Here's how the part is built. I have some questions about the finished solid (model axes, mm). A direction names the side the tool comes from. Coordinates: 2 decimals unless noted, no trailing zeros. Loops run counter-clockwise (first coordinate to the right, second up) from the corner with the lowest first, then second, coordinate; pieces in that order, holes last. Notation, with made-up numbers: M 64,84.25 L 84,84.25 A7 cw 84,94.25 Z; hole C -11,70.5 d2. An arc over 180 degrees is marked long. Use CSV: the item, a comma, the result in double quotes. Start each with the question number.
Q1. If we section it at A-A (z = 0): Please give me the cut outline in (x, y), and give its area (3 significant figures).
Q2. Which directions (+Z, -Z, +X, -X, +Y, -Y) give clear straight access to the entire face, cutting with the end or side of a thin tool? Please do faces 4 (the cylindrical face through (-14, 1, 0)), 5 (the flat face through (-13.67, 4.08, 7.9)), 6 (the flat face through (13.84, 4.08, 7.79)), 7 (the cylindrical face through (0, 4, -14)), 8 (the flat face through (-20, 4, 3)).
Q3. If we mould it in two halves opening along X, with no side actions, what happens to faces 1 (the cylindrical face through (16.05, 4.08, -0.08)), 2 (the flat face through (20, 4, -3)), 3 (the flat face through (-4, 0, -5))? For each: +X half, -X half, draft (parallel to the pull), parting line (faces both ways), or undercut.
Q4. If we section it at D-D (y = 1.05): Please give me the cut outline in (x, z), and give its area (3 significant figures).
Q5. For pin 1 Ø6 at (x, z) = (15.5, 15.5) entering from +Y, with a flat end and sliding along its axis, tell me the tip position at first contact or that it passes through.
Q6. If we section it at C-C (y = 3.65): Please give me the cut outline in (x, z), and give its area (3 significant figures).
Q7. Please list where these lines run through material, in increasing order: probe 1 along Z at (x, y) = (17, 1.3); probe 2 along Y at (x, z) = (-13.5, 15.5); probe 3 along Z at (x, y) = (2, 2.2). Write a range as [from, to].
Q8. If we section it at B-B (x = 0): Please give me the cut outline in (y, z), and give its area (3 significant figures).
from build123d import *

# Parameters (mm, degrees)
SKETCH_1_R          = 1.8
SKETCH_1_R_2        = 5
EXTRUDE_1_DEPTH     = 3
EXTRUDE_2_DEPTH     = 2.2
SKETCH_3_R          = 5
CUT_EXTRUDE_1_DEPTH = 2.2


with BuildPart() as part:
    # 草图1 → 凸台-拉伸1 (new body)
    with BuildSketch(Plane(origin=(0, 0, 0), x_dir=(1, 0, 0), z_dir=(0, 1, 0))):
        with BuildLine():
            Line((20, -3.872983346), (20, -15))
            ThreePointArc((20, -15), (18.535533906, -18.535533906), (15, -20))
            Line((15, -20), (-15, -20))
            ThreePointArc((-15, -20), (-18.535533906, -18.535533906), (-20, -15))
            Line((-20, -15), (-20, -3.872983346))
            ThreePointArc((-20, -3.872983346), (-14, 0), (-20, 3.872983346))
            Line((-20, 3.872983346), (-20, 15))
            ThreePointArc((-20, 15), (-18.535533906, 18.535533906), (-15, 20))
            Line((-15, 20), (15, 20))
            ThreePointArc((15, 20), (18.535533906, 18.535533906), (20, 15))
            Line((20, 15), (20, 3.872983346))
            ThreePointArc((20, 3.872983346), (14, 0), (20, -3.872983346))
        make_face()
        with Locations((-15.5, 15.5)):
            Circle(SKETCH_1_R, mode=Mode.SUBTRACT)
        with Locations((15.5, 15.5)):
            Circle(SKETCH_1_R, mode=Mode.SUBTRACT)
        with Locations((-15.5, -15.5)):
            Circle(SKETCH_1_R, mode=Mode.SUBTRACT)
        with Locations((15.5, -15.5)):
            Circle(SKETCH_1_R, mode=Mode.SUBTRACT)
        Circle(SKETCH_1_R_2, mode=Mode.SUBTRACT)
    extrude(amount=EXTRUDE_1_DEPTH)

    # 草图2 → 凸台-拉伸2 (add)
    with BuildSketch(Plane(origin=(0, 3, 0), x_dir=(1, 0, 0), z_dir=(0, 1, 0))):
        with BuildLine():
            Line((-20, 3.872983346), (-7.512267775, 11.81379841))
            ThreePointArc((-7.512267775, 11.81379841), (0, 14), (7.512267775, 11.81379841))
            Line((7.512267775, 11.81379841), (20, 3.872983346))
            Line((20, 3.872983346), (20, 1.333229163))
            ThreePointArc((20, 1.333229163), (16.05, 0), (20, -1.333229163))
            Line((20, -1.333229163), (20, -3.872983346))
            Line((20, -3.872983346), (7.512267775, -11.81379841))
            ThreePointArc((7.512267775, -11.81379841), (0, -14), (-7.512267775, -11.81379841))
            Line((-7.512267775, -11.81379841), (-20, -3.872983346))
            Line((-20, -3.872983346), (-20, -1.333229163))
            ThreePointArc((-20, -1.333229163), (-16.05, 0), (-20, 1.333229163))
            Line((-20, 1.333229163), (-20, 3.872983346))
        make_face()
    extrude(amount=EXTRUDE_2_DEPTH)

    # 草图3 → 切除-拉伸1 (cut)
    with BuildSketch(Plane.XZ.offset(-3)):
        Circle(SKETCH_3_R)
    extrude(amount=-CUT_EXTRUDE_1_DEPTH, mode=Mode.SUBTRACT)


solid = part.part
Results below:
1,outline,"M -16.05,3 L -14,3 L -14,0 L -5,0 L -5,5.2 L -16.05,5.2 Z; M 5,0 L 14,0 L 14,3 L 16.05,3 L 16.05,5.2 L 5,5.2 Z"
1,area,"103 mm^2"
2,face 4,"-Y"
2,face 5,"+Z, -X, +Y"
2,face 6,"+Z, +X, +Y"
2,face 7,"-Z, +Y"
2,face 8,"+Z, -Z, -X, +Y, -Y"
3,face 1,"undercut"
3,face 2,"+X half"
3,face 3,"draft"
4,outline,"M -20,-15 A5 ccw -15,-20 L 15,-20 A5 ccw 20,-15 L 20,-3.87 A4.25 cw long 20,3.87 L 20,15 A5 ccw 15,20 L -15,20 A5 ccw -20,15 L -20,3.87 A4.25 cw long -20,-3.87 Z; hole C -15.5,-15.5 d3.6; hole C -15.5,15.5 d3.6; hole C 0,0 d10; hole C 15.5,-15.5 d3.6; hole C 15.5,15.5 d3.6"
4,area,"1,370 mm^2"
5,pin 1,"y = 3"
6,outline,"M -20,-3.87 L -7.51,-11.81 A14 ccw 7.51,-11.81 L 20,-3.87 L 20,-1.33 A2.2 cw long 20,1.33 L 20,3.87 L 7.51,11.81 A14 ccw -7.51,11.81 L -20,3.87 L -20,1.33 A2.2 cw long -20,-1.33 Z; hole C 0,0 d10"
6,area,"684 mm^2"
7,probe 1,"[-19.58, -16.49], [-14.51, -4.06], [4.06, 14.51], [16.49, 19.58]"
7,probe 2,"[0, 3]"
7,probe 3,"[-20, -4.58], [4.58, 20]"
8,outline,"M 0,-20 L 3,-20 L 3,-14 L 5.2,-14 L 5.2,-5 L 0,-5 Z; M 0,5 L 5.2,5 L 5.2,14 L 3,14 L 3,20 L 0,20 Z"
8,area,"130 mm^2"
